CAD build for the part. Positions are in the model's coordinates, mm. A direction names the side the tool comes from. Round coordinates to 2 decimals unless told otherwise and drop trailing zeros. Loops run counter-clockwise (first coordinate to the right, second up) from the corner with the lowest first, then second, coordinate; pieces in that order, holes last. Notation, with made-up numbers: (43.25, 1) -> (65.25, 1) arc R23 ccw to (65.25, 26) -> close; hole circle Ø8 at (57, 2.25). An arc over 180 degrees is marked (long way). Answer as CSV lines item,"result".
```python
from build123d import *

# Parameters (mm, degrees)
F0_R     = 4
F0_R_2   = 3
F2_DEPTH = 9.1
F1_R     = 11.5
F3_DEPTH = 2
F4_R     = 4.5
F5_DEPTH = 2.5


with BuildPart() as f2:
    # F0 (on Front) → F2 (new body)
    with BuildSketch(Plane.XZ):
        Circle(F0_R)
        Circle(F0_R_2, mode=Mode.SUBTRACT)
    extrude(amount=F2_DEPTH)

    # F1 (on Front) → F3 (join)
    with BuildSketch(Plane.XZ):
        Circle(F1_R)
    extrude(amount=F3_DEPTH)

    # F4 (on Front) → F5 (join)
    with BuildSketch(Plane.XZ):
        Circle(F4_R)
    extrude(amount=F5_DEPTH)


solid = f2.part
```
Q1. Drop flat-ended pins along their axis: pin 1 Ø3 at (x, z) = (0.5, 1) entering from -Y; pin 2 Ø10 at (x, z) = (-1.5, -1) entering from -Y; pin 3 Ø5 at (x, y) = (4, -1.5) entering from -Z; pin 4 Ø1.5 at (y, z) = (-5.5, 2.5) entering from +X. Give the stop position or say it passes through.
Results:
pin 1,"y = -2.5"
pin 2,"y = -9.1"
pin 3,"z = -11.4"
pin 4,"x = 3.6"
Q2. Probe L1, parallel to X at y = -4.75, z = 0; L2, parallel to Y at x = -6.75, z = -5.5. List the from-to ranges inside material, lowest first. Write a range as [from, to].
Results:
L1,"[-4, -3], [3, 4]"
L2,"[-2, 0]"
Q3. Tool access for faces 4 (the cylindrical face through (-3, -6, 0)), 5 (the flat face through (0, 0, 0)): list every direction of +Z, -Z, +X, -X, +Y, -Y with a clear straight run to the whole face (end or side of a thin tool).
Results:
face 4,"-Y"
face 5,"+Z, -Z, +X, -X, +Y"
Q4. Slice it at C-C, the plane y = -6. Give the cut face in (x, z), and give its area (3 significant figures).
Results:
outline,"circle Ø8 at (0, 0); hole circle Ø6 at (0, 0)"
area,"22.0 mm2"
Q5. Slice it at D-D, the plane y = -1.25. Give the cut face in (x, z), and give its area (3 significant figures).
Results:
outline,"circle Ø23 at (0, 0)"
area,"415 mm2"
Q6. Slice it at B-B, the plane z = 0. Give the cut face in (x, y).
Results:
outline,"(-11.5, -2) -> (-4.5, -2) -> (-4.5, -2.5) -> (-4, -2.5) -> (-4, -9.1) -> (-3, -9.1) -> (-3, -2.5) -> (3, -2.5) -> (3, -9.1) -> (4, -9.1) -> (4, -2.5) -> (4.5, -2.5) -> (4.5, -2) -> (11.5, -2) -> (11.5, 0) -> (-11.5, 0) -> close"
Q7. Two-plate mould, pull along Z, no slides. Class faces 1 (the flat face through (1, -9.1, 3)), 2 (the cylindrical face through (-0.867, -5.754, -3.905)), 3 (the flat face through (0, -2.5, 0)): pulls with the +Z half, pulls with the -Z half, needs draft (parallel to the pull), parting line crosses it, or undercut.
Results:
face 1,"needs draft"
face 2,"parting line crosses it"
face 3,"undercut"
Q8. Slice it at A-A, the plane x = 0. Give the cut face in (y, z), and give its area (3 significant figures).
Results:
outline,"(-9.1, -4) -> (-2.5, -4) -> (-2.5, -4.5) -> (-2, -4.5) -> (-2, -11.5) -> (0, -11.5) -> (0, 11.5) -> (-2, 11.5) -> (-2, 4.5) -> (-2.5, 4.5) -> (-2.5, 4) -> (-9.1, 4) -> (-9.1, 3) -> (-2.5, 3) -> (-2.5, -3) -> (-9.1, -3) -> close"
area,"63.7 mm2"
